For this review, take the finished solid that the model builds, in its own axes (mm). A direction names the side the tool comes from. Round coordinates to 2 decimals unless told otherwise and drop trailing zeros. Order: outer loops, then holes, each group sorted by start corner. A loop starts at its lowest first (then second) coordinate and runs counter-clockwise, first axis right, second up. Notation, with made-up numbers: M -39.5,52 L -35.5,52 A17 ccw -35.5,57 Z; hole C -7,46 d4. An arc over 180 degrees is marked long. Answer as a JSON object with one key per item and string values.
from build123d import *

# Parameters (mm, degrees)
SKETCH_1_W          = 53
SKETCH_1_H          = 51
EXTRUDE_1_DEPTH     = 50
SKETCH_2_W          = 50
SKETCH_2_H          = 48
CUT_EXTRUDE_1_DEPTH = 50
CUT_EXTRUDE_2_DEPTH = 25
SKETCH_4_R          = 11.05
SKETCH_4_R_2        = 1.6
CUT_EXTRUDE_3_DEPTH = 50


with BuildPart() as part:
    # 草图1 → 凸台-拉伸1 (new body)
    with BuildSketch(Plane(origin=(0, 0, 0), x_dir=(0, 0, -1), z_dir=(1, 0, 0))):
        with Locations((26.5, 25.5)):
            Rectangle(SKETCH_1_W, SKETCH_1_H)
    extrude(amount=EXTRUDE_1_DEPTH)

    # 草图2 → 切除-拉伸1 (cut)
    with BuildSketch(Plane.ZY):
        with Locations((-25, 27)):
            Rectangle(SKETCH_2_W, SKETCH_2_H)
    extrude(amount=-CUT_EXTRUDE_1_DEPTH, mode=Mode.SUBTRACT)

    # 草图3 → 切除-拉伸2 (cut, symmetric)
    with BuildSketch(Plane(origin=(0, 3, 0), x_dir=(1, 0, 0), z_dir=(0, 1, 0))):
        with BuildLine():
            Line((7.9, 41), (7.9, 11))
            ThreePointArc((7.9, 11), (10, 8.9), (12.1, 11))
            Line((12.1, 11), (12.1, 41))
            ThreePointArc((12.1, 41), (10, 43.1), (7.9, 41))
        make_face()
        with BuildLine():
            Line((37.9, 41), (37.9, 11))
            ThreePointArc((37.9, 11), (40, 8.9), (42.1, 11))
            Line((42.1, 11), (42.1, 41))
            ThreePointArc((42.1, 41), (40, 43.1), (37.9, 41))
        make_face()
    extrude(amount=CUT_EXTRUDE_2_DEPTH, both=True, mode=Mode.SUBTRACT)

    # 草图4 → 切除-拉伸3 (cut)
    with BuildSketch(Plane.XY.offset(-50)):
        with Locations((25, 33)):
            Circle(SKETCH_4_R)
        with Locations((9.5, 45.5)):
            Circle(SKETCH_4_R_2)
        with Locations((40.5, 45.5)):
            Circle(SKETCH_4_R_2)
        with Locations((9.5, 14.5)):
            Circle(SKETCH_4_R_2)
        with Locations((40.5, 14.5)):
            Circle(SKETCH_4_R_2)
        Polygon((5.5, 51), (0, 45.5), (0, 51), align=None)
        Polygon((44.5, 51), (50, 45.5), (50, 51), align=None)
    extrude(amount=-CUT_EXTRUDE_3_DEPTH, mode=Mode.SUBTRACT)


solid = part.part
1) Mouldability with a two-part tool opening along Z and no side actions: class faces 1 (the cylindrical face through (8.32, 15.58, -51.48)), 2 (the flat face through (12.1, 1, -26)), 3 (the flat face through (25, 19, -53)), 4 (the flat face through (25, 21, -50)) as +Z half, -Z half, draft (parallel to the pull), parting line (faces both ways), or undercut.
Geometry check:
{"face 1": "draft", "face 2": "undercut", "face 3": "-Z half", "face 4": "+Z half"}
2) For L1, parallel to Y at x = 40.5, z = -51.2; L2, parallel to Y at x = 9, z = -52; L3, parallel to Z at x = 12.5, y = 28, list the stretches that pass through material, from the lowest coordinate up.
Geometry check:
{"L1": "y = 0 to 12.9, 16.1 to 43.9, 47.1 to 51", "L2": "y = 0 to 12.98, 16.02 to 43.98, 47.02 to 51", "L3": "z = -53 to -50"}
3) Add section B-B on x = 25. State the section outline as (y, z) points, and give its area (3 significant figures).
Geometry check:
{"outline": "M 0,-53 L 21.95,-53 L 21.95,-50 L 3,-50 L 3,0 L 0,0 Z; M 44.05,-53 L 51,-53 L 51,-50 L 44.05,-50 Z", "area": "237 mm²"}
4) Insertion check: P1, Ø6, axis at x = 19, y = 34, coming from the -Z side; P2, Ø6, axis at x = 21, z = -8, coming from the +Y side; P3, Ø3.5, axis at x = 9.5, y = 45.5, coming from the +Z side. Each pin has a flat end and moves straight along its axis. Give the tip position at first contact, or say it passes through.
Geometry check:
{"P1": "passes through", "P2": "stops at y = 3", "P3": "stops at z = -50"}
5) Add section C-C on y = 33. State the section outline as (x, z) points, and give its area (3 significant figures).
Geometry check:
{"outline": "M 0,-53 L 13.95,-53 L 13.95,-50 L 0,-50 Z; M 36.05,-53 L 50,-53 L 50,-50 L 36.05,-50 Z", "area": "83.7 mm²"}
6) Add section D-D on y = 14.5. State the section outline as (x, z) points, and give its area (3 significant figures).
Geometry check:
{"outline": "M 0,-53 L 7.9,-53 L 7.9,-50 L 0,-50 Z; M 11.1,-53 L 38.9,-53 L 38.9,-50 L 11.1,-50 Z; M 42.1,-53 L 50,-53 L 50,-50 L 42.1,-50 Z", "area": "131 mm²"}
7) Add section A-A on z = -26. State the section outline as (x, y) points.
Geometry check:
{"outline": "M 0,0 L 7.9,0 L 7.9,3 L 0,3 Z; M 12.1,0 L 37.9,0 L 37.9,3 L 12.1,3 Z; M 42.1,0 L 50,0 L 50,3 L 42.1,3 Z"}
8) Machinability: for faces 5 (the cylindrical face through (10, 1.5, -43.1)), 6 (the cylindrical face through (9.15, 43.94, -51.48)), which of the approach directions +Z, -Z, +X, -X, +Y, -Y give a long, thin tool a straight path to every point of the face, cutting with its end or side? Answer none if there is none.
Geometry check:
{"face 5": "+Y, -Y", "face 6": "+Z, -Z"}
